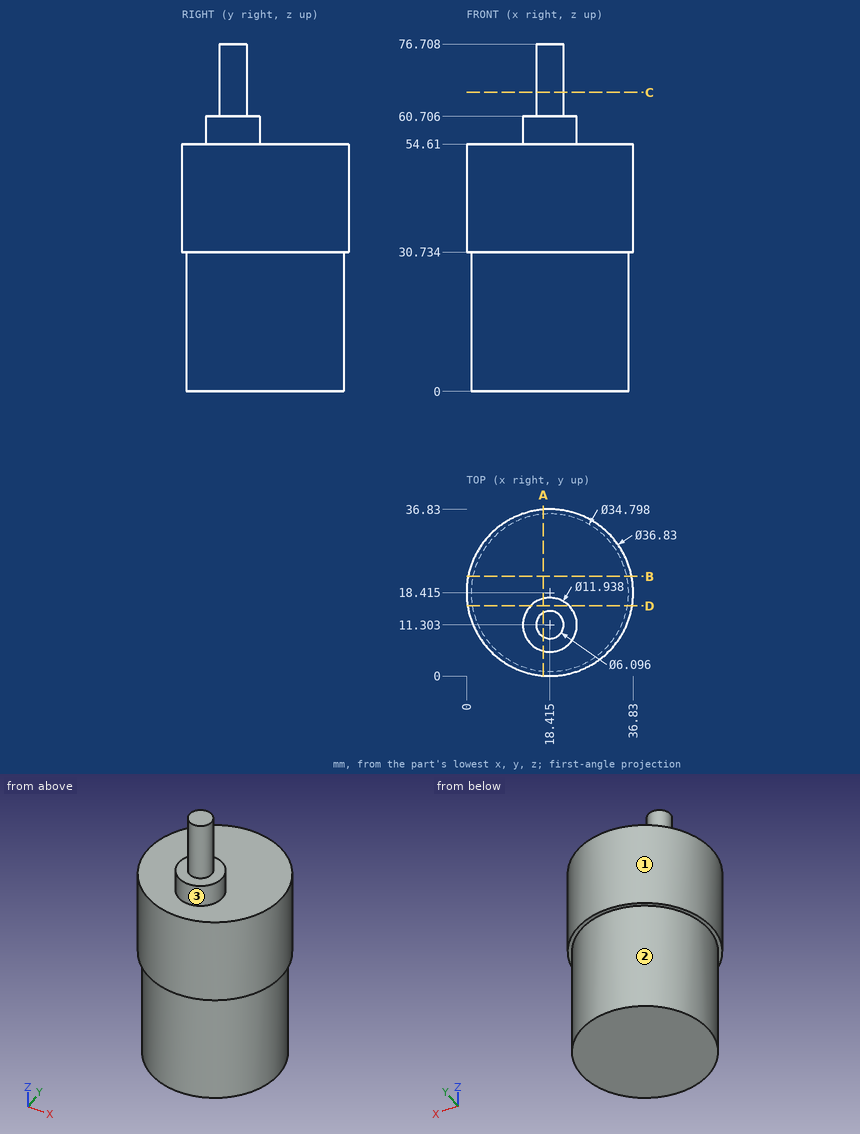
Can you work these out from the drawing? Everything is in mm from the part's minimum corner. A direction names the side the tool comes from. Give positions to 0.01 mm unless a question says otherwise; leave off trailing zeros. Loops run counter-clockwise (first coordinate to the right, second up) from the corner with the lowest first, then second, coordinate; pieces in that order, holes last. Notation, with made-up numbers: (-9.5, -26.5) -> (14.5, -26.5) arc R21 ccw to (14.5, 7.5) -> close; hole circle Ø6 at (75, 60). An arc over 180 degrees is marked (long way). Write item = value, one per line.
1) Suppose I cut it at A-A on x = 17. Write out the boundary of the cut face in (y, z), then the cut area to 3 significant figures.
Check result:
outline = (0.05, 30.73) -> (1.07, 30.73) -> (1.07, 0) -> (35.76, 0) -> (35.76, 30.73) -> (36.78, 30.73) -> (36.78, 54.61) -> (17.1, 54.61) -> (17.1, 60.71) -> (14, 60.71) -> (14, 76.71) -> (8.6, 76.71) -> (8.6, 60.71) -> (5.5, 60.71) -> (5.5, 54.61) -> (0.05, 54.61) -> close
area = 2,100 mm2
2) Suppose I cut it at D-D on y = 15.5. Write out the boundary of the cut face in (x, z).
Check result:
outline = (0.23, 30.73) -> (1.26, 30.73) -> (1.26, 0) -> (35.57, 0) -> (35.57, 30.73) -> (36.6, 30.73) -> (36.6, 54.61) -> (22.66, 54.61) -> (22.66, 60.71) -> (14.17, 60.71) -> (14.17, 54.61) -> (0.23, 54.61) -> close
3) I need wall thicknesses on L1, parallel to Z at x = 23.5, y = 35.5; L2, parallel to Z at x = 21.5, y = 32; L3, parallel to X at y = 11, z = 63.5. Which ranges of each line are inside material? Lowest first, please. Write a range as from..to.
Check result:
L1 = 30.73..54.61
L2 = 0..54.61
L3 = 15.38..21.45
4) Suppose I cut it at C-C on z = 66. Write out the boundary of the cut face in (x, y) (3 decimals), then the cut area to 3 significant figures.
Check result:
outline = circle Ø6.096 at (18.415, 11.303)
area = 29.2 mm2
5) Suppose I cut it at B-B on y = 22. Write out the boundary of the cut face in (x, z).
Check result:
outline = (0.35, 30.73) -> (1.39, 30.73) -> (1.39, 0) -> (35.44, 0) -> (35.44, 30.73) -> (36.48, 30.73) -> (36.48, 54.61) -> (0.35, 54.61) -> close
6) For the marked faces 1, 2 and 3, which set-ups out of +Z, -Z, +X, -X, +Y, -Y let a thin tool reach every point of the face, with its end or its side?
Check result:
face_1 = +Z, -Z
face_2 = -Z
face_3 = +Z
7) Will these pins go through, and if not, where does the flat tip stop? pin 1 (6 mm diameter, centred on x = 4.5, y = 28.5, fed in from +Z); pin 2 (12 mm diameter, centred on y = 10, z = 40.5, fed in from +X); pin 3 (4 mm diameter, centred on x = 10, z = 10.5, fed in from +Y); pin 4 (4 mm diameter, centred on y = 4.5, z = 66.5, fed in from -X).
Check result:
pin_1 = 54.61
pin_2 = 36.67
pin_3 = 34.59
pin_4 = through
